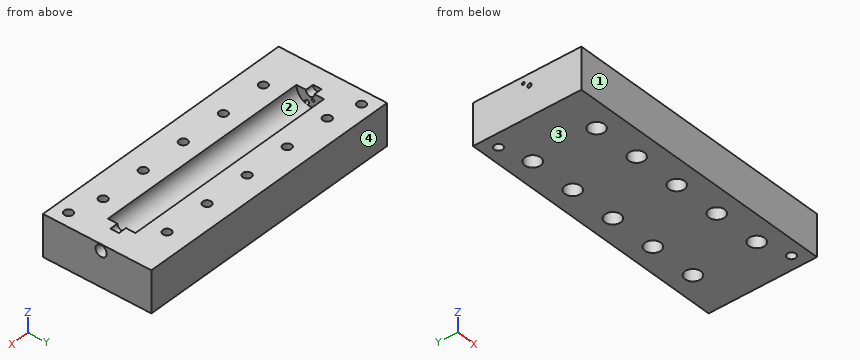
from build123d import *

# Parameters (mm, degrees)
SKIZZE2_W                            = 100
SKIZZE2_H                            = 39.364160046
AUFSATZ_LINEAR_AUSTRAGEN1_DEPTH      = 30
SCHNITT_LINEAR_AUSTRAGEN1_DEPTH      = 40
SCHNITT_LINEAR_AUSTRAGEN1_DEPTH_BACK = 40
SKIZZE10_R                           = 5
SKIZZE17_R                           = 1.55
SCHNITT_LINEAR_AUSTRAGEN2_DEPTH      = 3
SKIZZE24_R                           = 1.55
SCHNITT_LINEAR_AUSTRAGEN4_DEPTH      = 112.577493681
SKIZZE37_R                           = 0.736865544
SCHNITT_LINEAR_AUSTRAGEN9_DEPTH      = 112.577493681
SKIZZE40_R                           = 2.1
SCHNITT_LINEAR_AUSTRAGEN10_DEPTH     = 6
SKIZZE42_R                           = 0.75
SCHNITT_LINEAR_AUSTRAGEN12_DEPTH     = 10
SKIZZE46_R                           = 2.85
SCHNITT_LINEAR_AUSTRAGEN15_DEPTH     = 10
SCHNITT_LINEAR_START                 = -5
SCHNITT_LINEAR_AUSTRAGEN25_DEPTH     = 2.7
LINEARES_MUSTER1_COUNT               = 5
LINEARES_MUSTER1_PITCH               = 17
SPIEGELN2_COPY_1_SKETCH_R            = 2.85
SPIEGELN2_COPY_1_DEPTH               = 10
SPIEGELN2_COPY_2_SKETCH_R            = 2.85
SPIEGELN2_COPY_2_DEPTH               = 10
SPIEGELN2_COPY_3_SKETCH_R            = 2.85
SPIEGELN2_COPY_3_DEPTH               = 10
SPIEGELN2_COPY_4_SKETCH_R            = 2.85
SPIEGELN2_COPY_4_DEPTH               = 10
SPIEGELN2_START                      = -5
SPIEGELN2_COPY_5_DEPTH               = 2.7
SPIEGELN2_COPY_6_DEPTH               = 2.7
SPIEGELN2_COPY_7_DEPTH               = 2.7
SPIEGELN2_COPY_8_DEPTH               = 2.7
SKIZZE51_R                           = 1.55
SCHNITT_LINEAR_AUSTRAGEN26_DEPTH     = 112.577493681
SKIZZE55_R                           = 0.5
SCHNITT_LINEAR_AUSTRAGEN28_DEPTH     = 112.577493681
SKIZZE59_R                           = 2.05
SCHNITT_LINEAR_AUSTRAGEN30_DEPTH     = 5
FASE1_SIZE                           = 1
FASE2_SIZE                           = 1
ABSPALTEN3_SURFACE_1_BACK            = 112.577
ABSPALTEN3_SURFACE_1_DEPTH           = 225.154


with BuildPart() as part:
    # Skizze2 → Aufsatz-Linear austragen1 (new body)
    with BuildSketch(Plane.XY):
        with Locations((50, 19.682080023)):
            Rectangle(SKIZZE2_W, SKIZZE2_H)
    extrude(amount=AUFSATZ_LINEAR_AUSTRAGEN1_DEPTH)

    # Skizze10 → Schnitt-Linear austragen1 (cut, two sides: drawn at the far end of the back side and taken through both)
    with BuildSketch(Plane.ZY.offset(-50).offset(-SCHNITT_LINEAR_AUSTRAGEN1_DEPTH_BACK)):
        with Locations((14.945770016, 20.027045739)):
            Circle(SKIZZE10_R)
    extrude(amount=SCHNITT_LINEAR_AUSTRAGEN1_DEPTH + SCHNITT_LINEAR_AUSTRAGEN1_DEPTH_BACK, mode=Mode.SUBTRACT)

    # Skizze17 → Schnitt-Linear austragen2 (cut)
    with BuildSketch(Plane.ZY.offset(-90)):
        with Locations((14.945770016, 20.027045739)):
            Circle(SKIZZE17_R)
    schnitt_linear_austragen2 = extrude(amount=-SCHNITT_LINEAR_AUSTRAGEN2_DEPTH, mode=Mode.SUBTRACT)

    # Spiegeln1: Schnitt-Linear austragen2 across plane
    add(schnitt_linear_austragen2.mirror(Plane.ZY.offset(-50)), mode=Mode.SUBTRACT)

    # Skizze24 → Schnitt-Linear austragen4 (cut, through all)
    with BuildSketch(Plane.XY.offset(30)):
        with Locations((16, 31.364160046)):
            Circle(SKIZZE24_R)
        with Locations((33, 31.364160046)):
            Circle(SKIZZE24_R)
        with Locations((50, 31.364160046)):
            Circle(SKIZZE24_R)
        with Locations((67, 31.364160046)):
            Circle(SKIZZE24_R)
        with Locations((84, 31.364160046)):
            Circle(SKIZZE24_R)
    schnitt_linear_austragen4 = extrude(amount=-SCHNITT_LINEAR_AUSTRAGEN4_DEPTH, mode=Mode.SUBTRACT)

    # Skizze37 → Schnitt-Linear austragen9 (cut, through all)
    with BuildSketch(Plane(origin=(100, 0, 0), x_dir=(0, 0, -1), z_dir=(1, 0, 0))):
        with Locations((-18.924590299, 18.633559666)):
            Circle(SKIZZE37_R)
    extrude(amount=-SCHNITT_LINEAR_AUSTRAGEN9_DEPTH, mode=Mode.SUBTRACT)

    # Skizze40 → Schnitt-Linear austragen10 (cut)
    with BuildSketch(Plane(origin=(100, 0, 0), x_dir=(0, 0, -1), z_dir=(1, 0, 0))):
        with Locations((-18.924590299, 18.633559666)):
            Circle(SKIZZE40_R)
    extrude(amount=-SCHNITT_LINEAR_AUSTRAGEN10_DEPTH, mode=Mode.SUBTRACT)

    # Skizze42 → Schnitt-Linear austragen12 (cut)
    with BuildSketch(Plane.ZY):
        with Locations((10.86415918, 18.842582577)):
            Circle(SKIZZE42_R)
    extrude(amount=-SCHNITT_LINEAR_AUSTRAGEN12_DEPTH, mode=Mode.SUBTRACT)

    # Skizze46 → Schnitt-Linear austragen15 (cut)
    with BuildSketch(Plane(origin=(0, 0, 0), x_dir=(-1, 0, 0), z_dir=(0, 0, -1))):
        with Locations((-84, 31.364160046)):
            Circle(SKIZZE46_R)
    schnitt_linear_austragen15 = extrude(amount=-SCHNITT_LINEAR_AUSTRAGEN15_DEPTH, mode=Mode.SUBTRACT)

    # Skizze50 → Schnitt-Linear austragen25 (cut)
    with BuildSketch(Plane.XY.offset(30).offset(SCHNITT_LINEAR_START)):
        Polygon((81.15, 33.009608314), (81.15, 39.364160046), (86.85, 39.364160046), (86.85, 33.009608314), (86.85, 29.718711779), (84, 28.073263512), (81.15, 29.718711779), align=None)
    schnitt_linear_austragen25 = extrude(amount=-SCHNITT_LINEAR_AUSTRAGEN25_DEPTH, mode=Mode.SUBTRACT)

    # Lineares Muster1: Schnitt-Linear austragen15, Schnitt-Linear austragen25 ×5
    with Locations(*[(-i * LINEARES_MUSTER1_PITCH, 0, 0) for i in range(1, LINEARES_MUSTER1_COUNT)]):
        add(schnitt_linear_austragen15, mode=Mode.SUBTRACT)
        add(schnitt_linear_austragen25, mode=Mode.SUBTRACT)

    # Spiegeln2: Schnitt-Linear austragen15, Schnitt-Linear austragen25 across plane
    add(schnitt_linear_austragen15.mirror(Plane.ZX.offset(19.764160046)), mode=Mode.SUBTRACT)
    add(schnitt_linear_austragen25.mirror(Plane.ZX.offset(19.764160046)), mode=Mode.SUBTRACT)

    # Spiegeln2 copy 1 sketch → Spiegeln2 copy 1 (cut)
    with BuildSketch(Plane(origin=(-17, 39.528320093, 0), x_dir=(-1, 0, 0), z_dir=(0, 0, -1))):
        with Locations((-84, -31.364160046)):
            Circle(SPIEGELN2_COPY_1_SKETCH_R)
    extrude(amount=-SPIEGELN2_COPY_1_DEPTH, mode=Mode.SUBTRACT)

    # Spiegeln2 copy 2 sketch → Spiegeln2 copy 2 (cut)
    with BuildSketch(Plane(origin=(-34, 39.528320093, 0), x_dir=(-1, 0, 0), z_dir=(0, 0, -1))):
        with Locations((-84, -31.364160046)):
            Circle(SPIEGELN2_COPY_2_SKETCH_R)
    extrude(amount=-SPIEGELN2_COPY_2_DEPTH, mode=Mode.SUBTRACT)

    # Spiegeln2 copy 3 sketch → Spiegeln2 copy 3 (cut)
    with BuildSketch(Plane(origin=(-51, 39.528320093, 0), x_dir=(-1, 0, 0), z_dir=(0, 0, -1))):
        with Locations((-84, -31.364160046)):
            Circle(SPIEGELN2_COPY_3_SKETCH_R)
    extrude(amount=-SPIEGELN2_COPY_3_DEPTH, mode=Mode.SUBTRACT)

    # Spiegeln2 copy 4 sketch → Spiegeln2 copy 4 (cut)
    with BuildSketch(Plane(origin=(-68, 39.528320093, 0), x_dir=(-1, 0, 0), z_dir=(0, 0, -1))):
        with Locations((-84, -31.364160046)):
            Circle(SPIEGELN2_COPY_4_SKETCH_R)
    extrude(amount=-SPIEGELN2_COPY_4_DEPTH, mode=Mode.SUBTRACT)

    # Spiegeln2 copy 5 sketch → Spiegeln2 copy 5 (cut)
    with BuildSketch(Plane(origin=(-17, 39.528320093, 30), x_dir=(1, 0, 0), z_dir=(0, 0, 1)).offset(SPIEGELN2_START)):
        Polygon((81.15, -33.009608314), (81.15, -39.364160046), (86.85, -39.364160046), (86.85, -33.009608314), (86.85, -29.718711779), (84, -28.073263512), (81.15, -29.718711779), align=None)
    extrude(amount=-SPIEGELN2_COPY_5_DEPTH, mode=Mode.SUBTRACT)

    # Spiegeln2 copy 6 sketch → Spiegeln2 copy 6 (cut)
    with BuildSketch(Plane(origin=(-34, 39.528320093, 30), x_dir=(1, 0, 0), z_dir=(0, 0, 1)).offset(SPIEGELN2_START)):
        Polygon((81.15, -33.009608314), (81.15, -39.364160046), (86.85, -39.364160046), (86.85, -33.009608314), (86.85, -29.718711779), (84, -28.073263512), (81.15, -29.718711779), align=None)
    extrude(amount=-SPIEGELN2_COPY_6_DEPTH, mode=Mode.SUBTRACT)

    # Spiegeln2 copy 7 sketch → Spiegeln2 copy 7 (cut)
    with BuildSketch(Plane(origin=(-51, 39.528320093, 30), x_dir=(1, 0, 0), z_dir=(0, 0, 1)).offset(SPIEGELN2_START)):
        Polygon((81.15, -33.009608314), (81.15, -39.364160046), (86.85, -39.364160046), (86.85, -33.009608314), (86.85, -29.718711779), (84, -28.073263512), (81.15, -29.718711779), align=None)
    extrude(amount=-SPIEGELN2_COPY_7_DEPTH, mode=Mode.SUBTRACT)

    # Spiegeln2 copy 8 sketch → Spiegeln2 copy 8 (cut)
    with BuildSketch(Plane(origin=(-68, 39.528320093, 30), x_dir=(1, 0, 0), z_dir=(0, 0, 1)).offset(SPIEGELN2_START)):
        Polygon((81.15, -33.009608314), (81.15, -39.364160046), (86.85, -39.364160046), (86.85, -33.009608314), (86.85, -29.718711779), (84, -28.073263512), (81.15, -29.718711779), align=None)
    extrude(amount=-SPIEGELN2_COPY_8_DEPTH, mode=Mode.SUBTRACT)

    # Spiegeln3: Schnitt-Linear austragen4 across plane
    add(schnitt_linear_austragen4.mirror(Plane.ZX.offset(19.764160046)), mode=Mode.SUBTRACT)

    # Skizze51 → Schnitt-Linear austragen26 (cut, through all)
    with BuildSketch(Plane.XY.offset(30)):
        with Locations((5, 34.364160046)):
            Circle(SKIZZE51_R)
        with Locations((95, 5)):
            Circle(SKIZZE51_R)
    extrude(amount=-SCHNITT_LINEAR_AUSTRAGEN26_DEPTH, mode=Mode.SUBTRACT)

    # Skizze55 → Schnitt-Linear austragen28 (cut, through all)
    with BuildSketch(Plane(origin=(100, 0, 0), x_dir=(0, 0, -1), z_dir=(1, 0, 0))):
        with Locations((-12.633679338, 21.083160509)):
            Circle(SKIZZE55_R)
    extrude(amount=-SCHNITT_LINEAR_AUSTRAGEN28_DEPTH, mode=Mode.SUBTRACT)

    # Skizze59 → Schnitt-Linear austragen30 (cut)
    with BuildSketch(Plane(origin=(100, 0, 0), x_dir=(0, 0, -1), z_dir=(1, 0, 0))):
        with Locations((-12.633679338, 21.083160509)):
            Circle(SKIZZE59_R)
    extrude(amount=-SCHNITT_LINEAR_AUSTRAGEN30_DEPTH, mode=Mode.SUBTRACT)

    # Fase1
    fase1_edges = [part.edges().sort_by_distance(p)[0] for p in [
        (94, 18.633559666, 19.661455843),
    ]]
    chamfer(fase1_edges, length=FASE1_SIZE)

    # Fase2
    fase2_edges = [part.edges().sort_by_distance(p)[0] for p in [
        (95, 21.083160509, 13.133679338),
    ]]
    chamfer(fase2_edges, length=FASE2_SIZE)

    # Abspalten3: cut with a surface, the side behind it stays
    # Abspalten3 surface: a surface, the sketch's curves swept straight by 225.154 mm
    with BuildLine(Plane(origin=(100, 0, 0), x_dir=(0, 0, -1), z_dir=(1, 0, 0)).offset(-ABSPALTEN3_SURFACE_1_BACK), mode=Mode.PRIVATE) as abspalten3_surface_1_path:
        Line((-15, 39.364160046), (0, 39.364160046))
        Line((0, 39.364160046), (0, 0))
        Line((0, 0), (-15, 0))
        Line((-15, 0), (-15, 39.364160046))
    abspalten3_surface_1 = Shell.extrude(abspalten3_surface_1_path.wire(), (1 * ABSPALTEN3_SURFACE_1_DEPTH, 0 * ABSPALTEN3_SURFACE_1_DEPTH, 0 * ABSPALTEN3_SURFACE_1_DEPTH))
    split(bisect_by=abspalten3_surface_1, keep=Keep.BOTTOM)


solid = part.part
Work out the finished part from the listing and answer in its coordinate system (mm). Face numbers are marked on the shaded views. Coordinates: 2 decimals unless noted, no trailing zeros. Write each loop counter-clockwise with the first axis right and the second up, starting at its lowest first coordinate (ties: lowest second). Pieces come first, ordered by that corner, then holes. Notation, with made-up numbers: M 1,50.5 L 26,50.5 A15 cw 26,55.5 Z; hole C 39,64.5 d6. An arc over 180 degrees is marked long. Use one line per item in the form item = value. Start each with the question number.
1. Straight lines are drawn through the part: probe 1 along X at (y, z) = (8.5, 0.75); probe 2 along X at (y, z) = (21, 10.25); probe 3 along X at (y, z) = (34.5, 8.5). For each, find the intervals that lie inside material, in ascending order. Write a range as from..to.
2. The mould has two halves that part along Y. Classify the marked faces 1, 2, 3 and 4: released by +Y, released by -Y, zero draft, split by the parting line, or undercut.
3. The part is cut by section C-C (x = 33). Give the vertices of the cut face in (y, z).
4. The part is cut by section A-A (x = 5). Give the vertices of the cut face in (y, z).
5. The part is cut by section B-B (z = 7.25). Give the number of separate pieces and of enclosed holes in the cut face, plus the area to 3 significant figures.
6. Each of these flat-tipped pins is pushed along its axis until it touches: P1, Ø6.5, axis at x = 16.5, y = 30.5, coming from the -Z side; P2, Ø1.7, axis at x = 67.5, y = 8.5, coming from the -Z side; P3, Ø3, axis at x = 32.5, y = 30.5, coming from the -Z side. Where does it stop, or does it pass through?
7. The part is cut by section D-D (y = 16). Give the vertices of the cut face in (x, z), plus the area to 3 significant figures.
Evaluation:
q1.probe_1 = 0..13.17, 18.83..30.17, 35.83..47.17, 52.83..64.17, 69.83..81.17, 86.83..100
q1.probe_2 = 0..10, 90..100
q1.probe_3 = 0..3.46, 6.54..100
q2.face_1 = released by -Y
q2.face_2 = undercut
q2.face_3 = zero draft
q2.face_4 = released by +Y
q3.outline = M 0,0 L 5.31,0 L 5.31,10 L 6.61,10 L 6.61,15 L 0,15 Z; M 9.71,10 L 11.01,10 L 11.01,0 L 28.51,0 L 28.51,10 L 29.81,10 L 29.81,15 L 25.03,15 A5 cw long 15.03,15 L 9.71,15 Z; M 32.91,10 L 34.21,10 L 34.21,0 L 39.36,0 L 39.36,15 L 32.91,15 Z
q4.outline = M 0,0 L 32.81,0 L 32.81,15 L 0,15 Z; M 35.91,0 L 39.36,0 L 39.36,15 L 35.91,15 Z; hole C 18.84,10.86 d1.5; hole C 21.08,12.63 d1
q5.separate_pieces = 1
q5.enclosed_holes = 12
q5.area = 3,670 mm^2
q6.P1 = 0
q6.P2 = through
q6.P3 = 10
q7.outline = M 0,0 L 100,0 L 100,15 L 90,15 L 90,11.98 L 10,11.98 L 10,15 L 0,15 Z
q7.area = 1,260 mm^2
